Here's how the part is built. I have some questions about the finished solid (model axes, mm). A direction names the side the tool comes from. Coordinates: 2 decimals unless noted, no trailing zeros. Write each loop counter-clockwise with the first axis right and the second up, starting at its lowest first coordinate (ties: lowest second). Pieces come first, ordered by that corner, then holes. Notation, with made-up numbers: (-0.5, -38) - (54.5, -38) arc R15 ccw to (54.5, -21) - close; hole circle Ø9 at (-14, 35.25). An arc over 180 degrees is marked (long way). Answer in a Markdown table with one row per item. Add a question column.
Item 1: I'm going to push flat-ended pins straight in: pin 1 (11.5 mm diameter, centred on x = 17.5, y = 0, fed in from +Z); pin 2 (1.5 mm diameter, centred on x = -60.5, z = -1, fed in from -Y); pin 3 (6 mm diameter, centred on x = -131.5, z = -2.5, fed in from +Y); pin 4 (3 mm diameter, centred on x = -387, z = -9.5, fed in from +Y). Where does each tip first touch, or does it pass through?
Item 2: Imagine slicing it at A-A (z = 0). Please give me the cut outline in (x, y), plus the area to 3 significant figures.
Item 3: Imagine slicing it at B-B (x = -761.5). Please give me the cut outline in (y, z).
Item 4: If I drill on probe 1 along X at (y, z) = (0, 3); probe 2 along Y at (x, z) = (17.5, 0); probe 3 along Z at (x, y) = (-78, -0.5), over which ranges is the centre line in solid material (lowest first)? Write a range as from..to.
Item 5: Which directions (+Z, -Z, +X, -X, +Y, -Y) give clear straight access to the entire face, cutting with the end or side of a thin tool? Please do faces 1 (the face through (-419.05, 0.33, 7.493)), 2 (the face through (17.255, -6.703, -16.166)).
from build123d import *

# Parameters (mm, degrees)
SKETCH1_R               = 7.5
BOSS_EXTRUDE1_DEPTH     = 850
SKETCH2_R               = 17.5
BOSS_EXTRUDE2_DEPTH     = 35
SKETCH3_R               = 5
CUT_EXTRUDE2_DEPTH      = 18.5
CUT_EXTRUDE2_DEPTH_BACK = 18.5


with BuildPart() as part:
    # Sketch1 → Boss-Extrude1 (new body)
    with BuildSketch(Plane(origin=(0, 0, 0), x_dir=(0, 0, -1), z_dir=(1, 0, 0))):
        Circle(SKETCH1_R)
    extrude(amount=-BOSS_EXTRUDE1_DEPTH)

    # Sketch2 → Boss-Extrude2 (add)
    with BuildSketch(Plane(origin=(0, 0, 0), x_dir=(0, 0, -1), z_dir=(1, 0, 0))):
        Circle(SKETCH2_R)
    extrude(amount=BOSS_EXTRUDE2_DEPTH)

    # Sketch3 → Cut-Extrude2 (cut, two sides)
    with BuildSketch(Plane.XY) as cut_extrude2_sk:
        with Locations((17.5, 0)):
            Circle(SKETCH3_R)
    extrude(amount=CUT_EXTRUDE2_DEPTH, mode=Mode.SUBTRACT)
    extrude(cut_extrude2_sk.sketch, amount=-CUT_EXTRUDE2_DEPTH_BACK, mode=Mode.SUBTRACT)


solid = part.part
Here are the results:
| question | item | result |
|---|---|---|
| 1 | pin 1 | stops at z = 17.5 |
| 1 | pin 2 | stops at y = -7.5 |
| 1 | pin 3 | stops at y = 7.5 |
| 1 | pin 4 | passes through |
| 2 | outline | (-850, -7.5) - (0, -7.5) - (0, -17.5) - (35, -17.5) - (35, 17.5) - (0, 17.5) - (0, 7.5) - (-850, 7.5) - close; hole circle Ø10 at (17.5, 0) |
| 2 | area | 13,900 mm2 |
| 3 | outline | circle Ø15 at (0, 0) |
| 4 | probe 1 | x = -850..12.5, 22.5..35 |
| 4 | probe 2 | y = -17.5..-5, 5..17.5 |
| 4 | probe 3 | z = -7.48..7.48 |
| 5 | face 1 | -X |
| 5 | face 2 | +X, -X |
